Design review of the part built by this model. Coordinates are the model's own, in mm. Face numbers are marked on the shaded views. A direction names the side the tool comes from. Round coordinates to 2 decimals unless told otherwise and drop trailing zeros. Order: outer loops, then holes, each group sorted by start corner. A loop starts at its lowest first (then second) coordinate and runs counter-clockwise, first axis right, second up. Notation, with made-up numbers: M 30,24.25 L 85,24.25 A16 cw 85,41.25 Z; hole C 13,16 d4. An arc over 180 degrees is marked long. Write each question's results on one line, items separated by ' | '. Start each with the question number.
Item 1: Take a section at D-D, the plane y = 7. Write out the cut boundary in (x, z).
Item 2: Take a section at C-C, the plane z = 1. Count the separate pieces of the cut face and the enclosed holes in it, plus the area to 3 significant figures.
Item 3: Take a section at B-B, the plane x = 0. Write out the cut boundary in (y, z), plus the area to 3 significant figures.
Item 4: The part is to be moulded in two halves that separate along X. For the marked faces 6, 7 and 8, say which applies: +X half, -X half, draft (parallel to the pull), parting line (faces both ways), or undercut.
Item 5: Clearance check with flat-ended pins moving along their axes: pin 1 (5 mm diameter, centred on x = -23.8, z = -11.72, fed in from -Y); pin 2 (4 mm diameter, centred on x = -0.5, y = 22.5, fed in from -Z); pin 3 (14.5 mm diameter, centred on x = -4.5, y = 14.5, fed in from +Z); pin 4 (4 mm diameter, centred on x = -21.5, z = 5.5, fed in from +Y). State where each tip first meets the part, or that it passes through.
Item 6: Wall thickness on line 1 (X direction, y = 20.75, z = 0); line 2 (X direction, y = 21, z = 5); line 3 (Z direction, x = 10, y = 15.5): over which ranges is each line inside the solid? List them lowest first. Write a range as [from, to].
Item 7: Machinability: for the marked faces 1, 2, 3, 4 and 5, which of the approach directions +Z, -Z, +X, -X, +Y, -Y give a long, thin tool a straight path to every point of the face, cutting with its end or side? Answer none if there is none.
Item 8: Take a section at A-A, the plane y = 14.5. Write out the cut boundary in (x, z), plus the area to 3 significant figures.
Autodesk Fusion 360 part; units mm, degrees
sketch "Sketch1" plane through (0, 0, 0) normal (0, 1, 0) x (1, 0, 0)
  line L0 (29, 16) -> (-29, 16)
  line L1 (-29, 16) -> (-29, -16)
  line L2 (-29, -16) -> (29, -16)
  line L3 (29, -16) -> (29, 16)
  line L4 (23.8029, 11.7183) -> (-23.8029, 11.7183) construction
  line L5 (-23.8029, 11.7183) -> (-23.8029, -11.7183) construction
  line L6 (-23.8029, -11.7183) -> (23.8029, -11.7183) construction
  line L7 (23.8029, -11.7183) -> (23.8029, 11.7183) construction
  line L8 (23.8029, 11.7183) -> (-23.8029, -11.7183) construction
  line L9 (-23.8029, 11.7183) -> (23.8029, -11.7183) construction
  circle A0 centre (-23.8029, 11.7183) radius 1.55
  circle A1 centre (23.8029, 11.7183) radius 1.55
  circle A2 centre (23.8029, -11.7183) radius 1.55
  circle A3 centre (-23.8029, -11.7183) radius 1.55
  line L10 (-10, 0) -> (10, 0) construction
  circle A4 centre (-10, 0) radius 8.5
  circle A5 centre (10, 0) radius 8.5
  line L11 (0, 11.7183) -> (0, 16) construction
  dimension "d2" = 32
  dimension "d4" = 3.1
  dimension "d5" = 17
  dimension "d6" = 20
  dimension "d7" = 58
extrude "Extrude1" add sketch "Sketch1" along normal blind 5
sketch "Sketch2" plane through (0, 5, 0) normal (0, 1, 0) x (-1, 0, 0)
  circle A0 centre (-23.8029, -11.7183) radius 1.55
  circle A1 centre (23.8029, -11.7183) radius 1.55
  circle A2 centre (-23.8029, 11.7183) radius 1.55
  circle A3 centre (23.8029, 11.7183) radius 1.55
  circle A4 centre (10, 0) radius 8.5
  circle A5 centre (-10, 0) radius 8.5
  line L0 (-29, 16) -> (-29, -16)
  line L1 (-29, -16) -> (29, -16)
  line L2 (29, -16) -> (29, 16)
  line L3 (29, 16) -> (-29, 16)
  line L4 (10, 12) -> (-10, 12)
  arc A6 (-10, 12) -> (-10, -12) centre (-10, 0) ccw
  line L5 (-10, -12) -> (10, -12)
  arc A7 (10, -12) -> (10, 12) centre (10, 0) ccw
  line L6 (10, 0) -> (-10, 0) construction
  dimension "d10" = 20
  dimension "d11" = 12
extrude "Extrude2" add sketch "Sketch2" along normal blind 24 contours L4 A6 L5 A7
fillet "Fillet1" radius 5 4 edges at (-29, 2.5, 16) (-29, 2.5, -16) (29, 2.5, -16) (29, 2.5, 16)
fillet "Fillet2" radius 3 4 faces at (-3.3333, 13, 12) (20.0803, 13, -6.5106) (3.3333, 13, -12) (-17.2457, 21, -9.5656)
sketch "Sketch3" plane through (0, 29, 0) normal (0, 1, 0) x (-1, 0, 0)
  circle A0 centre (-10, 0) radius 8.5
  circle A1 centre (10, 0) radius 8.5
  line L0 (10, 9) -> (-10, 9)
  arc A2 (-10, 9) -> (-10, -9) centre (-10, 0) ccw
  line L1 (-10, -9) -> (10, -9)
  arc A3 (10, -9) -> (10, 9) centre (10, 0) ccw
  arc A4 (1.2397, 5.6527) -> (-1.2397, 5.6527) centre (0, 5) ccw
  arc A5 (1.2397, 5.6527) -> (2.1245, 6.1185) centre (1.6821, 5.8856) ccw
  arc A6 (2.1245, 6.1185) -> (-2.1245, 6.1185) centre (0, 5) ccw
  arc A7 (-2.1245, 6.1185) -> (-1.2397, 5.6527) centre (-1.6821, 5.8856) ccw
  arc A8 (1.6821, 5.8856) -> (-1.6821, 5.8856) centre (0, 5) ccw construction
  line L2 (0, 5) -> (0, 0) construction
  line L3 (1.6821, 5.8856) -> (-1.6821, 5.8856) construction
  dimension "d18" = 0.5
  dimension "d19" = 5
extrude "Extrude3" cut sketch "Sketch3" against normal blind 1 contours A4 A5 A6 A7
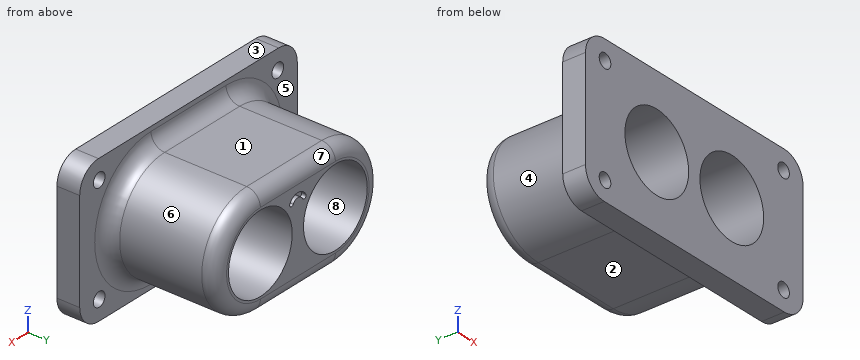
Results list:
1) outline: M -10,-12.17 L 10,-12.17 A12.17 ccw 10,12.17 L -10,12.17 A12.17 ccw Z; hole C -10,0 d17; hole C 10,0 d17
2) separate pieces: 3 | enclosed holes: 0 | area: 365 mm²
3) outline: M 0,-16 L 5,-16 L 5,-15 A3 cw 8,-12 L 26,-12 A3 ccw 29,-9 L 29,6.4 L 28,6.4 L 28,7.4 L 29,7.4 L 29,9 A3 ccw 26,12 L 8,12 A3 cw 5,15 L 5,16 L 0,16 Z | area: 735 mm²
4) face 6: +X half | face 7: draft | face 8: undercut
5) pin 1: y = 0 | pin 2: z = -12 | pin 3: z = 12.1 | pin 4: y = 28.44
6) line 1: [-22, -18.5], [-1.5, 1.5], [18.5, 22] | line 2: [-20.91, -16.87], [-3.13, 3.13], [16.87, 20.91] | line 3: [-12, -8.5], [8.5, 12]
7) face 1: +Z, +X, -X, +Y | face 2: -Z, +X, -X, +Y | face 3: +Z, +X, -X, +Y, -Y | face 4: -X, +Y | face 5: +Y
8) outline: M -10,-12 L 10,-12 A12 ccw 10,12 L -10,12 A12 ccw Z; hole C -10,0 d17; hole C 10,0 d17 | area: 478 mm²
